Job drawing, mm, ordinate dimensions from the low corner. One solid piece. A direction names the side the tool comes from. Give positions to 0.01 mm unless a question says otherwise; leave off trailing zeros. Order: outer loops, then holes, each group sorted by start corner. A loop starts at its lowest first (then second) coordinate and runs counter-clockwise, first axis right, second up. Notation, with made-up numbers: (21, -8) - (43, -8) arc R23 ccw to (43, 26) - close; hole circle Ø1 at (22.5, 52). An arc over 180 degrees is marked (long way). Use a Markdown table: item, result. Add a question column.
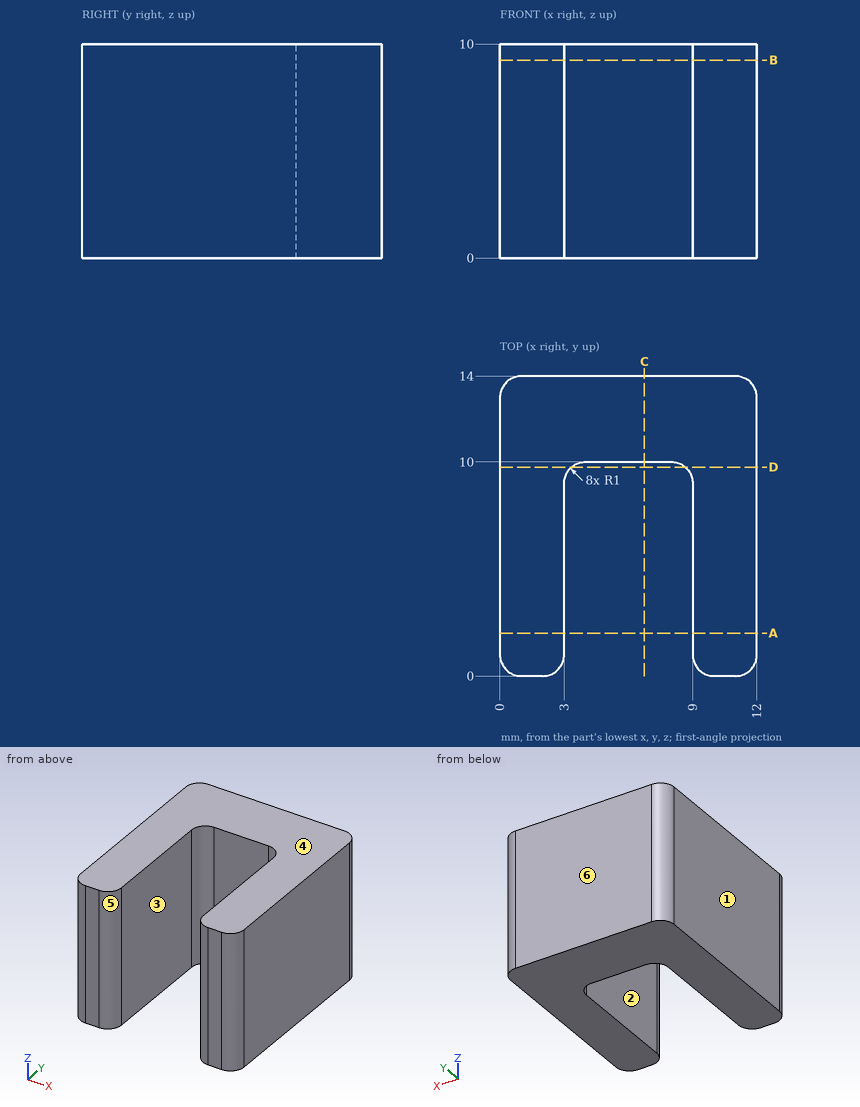
1. Cut at D-D (y = 9.75). Write the cut outline in (x, z), plus the area to 3 significant figures.
2. Pin check, flat tip, straight feed: P1, Ø3, axis at x = 7, z = 5, coming from the -Y side. Stop position of the tip, or through.
3. Drill centre lines: probe 1 along X at (y, z) = (5, 3.75); probe 2 along X at (y, z) = (0.5, 8); probe 3 along Y at (x, z) = (4.25, 2). Where is each one in solid material? Low to high. Write a range as [from, to].
4. Cut at C-C (x = 6.75). Write the cut outline in (y, z).
5. Cut at B-B (z = 9.25). Write the cut outline in (x, y), plus the area to 3 significant figures.
6. Tool access for the marked faces 5 and 6: list every direction of +Z, -Z, +X, -X, +Y, -Y with a clear straight run to the whole face (end or side of a thin tool).
7. Mould opens along X. For the marked faces 1, 2, 3 and 4 say: released by +X, released by -X, zero draft, split by the parting line, or undercut.
8. Cut at A-A (y = 2). Write the cut outline in (x, z).
Responses:
| question | item | result |
|---|---|---|
| 1 | outline | (0, 0) - (3.34, 0) - (3.34, 10) - (0, 10) - close; (8.66, 0) - (12, 0) - (12, 10) - (8.66, 10) - close |
| 1 | area | 66.8 mm² |
| 2 | P1 | stops at y = 9.87 |
| 3 | probe 1 | x = [0, 3], [9, 12] |
| 3 | probe 2 | x = [0.13, 2.87], [9.13, 11.87] |
| 3 | probe 3 | y = [10, 14] |
| 4 | outline | (10, 0) - (14, 0) - (14, 10) - (10, 10) - close |
| 5 | outline | (0, 1) arc R1 ccw to (1, 0) - (2, 0) arc R1 ccw to (3, 1) - (3, 9) arc R1 cw to (4, 10) - (8, 10) arc R1 cw to (9, 9) - (9, 1) arc R1 ccw to (10, 0) - (11, 0) arc R1 ccw to (12, 1) - (12, 13) arc R1 ccw to (11, 14) - (1, 14) arc R1 ccw to (0, 13) - close |
| 5 | area | 107 mm² |
| 6 | face 5 | +Z, -Z, -Y |
| 6 | face 6 | +Z, -Z, +X, -X, +Y |
| 7 | face 1 | released by -X |
| 7 | face 2 | undercut |
| 7 | face 3 | undercut |
| 7 | face 4 | zero draft |
| 8 | outline | (0, 0) - (3, 0) - (3, 10) - (0, 10) - close; (9, 0) - (12, 0) - (12, 10) - (9, 10) - close |
